from build123d import *

# Parameters (mm, degrees)
F0_W           = 116
F0_H           = 90
F1_DEPTH       = 15
F2_SIZE        = 0.5
F5_D           = 3
F5_DEPTH       = 8
F5_TIP         = 0.9012909285
F6_D           = 4.2
F6_DEPTH       = 13
F6_TIP         = 1.2618073
F7_D           = 5.5
F7_CBORE_D     = 10
F7_CBORE_DEPTH = 6.5


with BuildPart() as f1:
    # F0 (on Top) → F1 (new body)
    with BuildSketch(Plane.XY):
        with Locations((58, 45)):
            Rectangle(F0_W, F0_H)
    extrude(amount=F1_DEPTH)

    # F2
    f2_edges = [f1.edges().sort_by_distance(p)[0] for p in [
        (0, 45, 15),
        (58, 0, 15),
        (116, 45, 15),
        (58, 90, 15),
        (0, 45, 0),
        (58, 0, 0),
        (116, 45, 0),
        (58, 90, 0),
        (0, 0, 7.5),
        (116, 0, 7.5),
        (116, 90, 7.5),
        (0, 90, 7.5),
    ]]
    chamfer(f2_edges, length=F2_SIZE)

    # F5
    with Locations(Plane.XY.offset(15)):
        with Locations((101, 81), (31, 46), (13, 34), (83, 30)):
            Hole(F5_D / 2, depth=F5_DEPTH)
            with Locations((0, 0, -(F5_DEPTH + F5_TIP / 2))):  # 118° drill point
                Cone(0, F5_D / 2, F5_TIP, mode=Mode.SUBTRACT)

    # F6
    with Locations(Plane(origin=(0, 0, 0), x_dir=(1, 0, 0), z_dir=(0, 0, -1))):
        with Locations((105, -45), (11, -45)):
            Hole(F6_D / 2, depth=F6_DEPTH)
            with Locations((0, 0, -(F6_DEPTH + F6_TIP / 2))):  # 118° drill point
                Cone(0, F6_D / 2, F6_TIP, mode=Mode.SUBTRACT)

    # F7 (through all)
    with Locations(Plane(origin=(0, 0, 0), x_dir=(1, 0, 0), z_dir=(0, 0, -1))):
        with Locations((93.5, -61), (93.5, -31), (22, -40)):
            CounterBoreHole(F7_D / 2, F7_CBORE_D / 2, F7_CBORE_DEPTH)


solid = f1.part
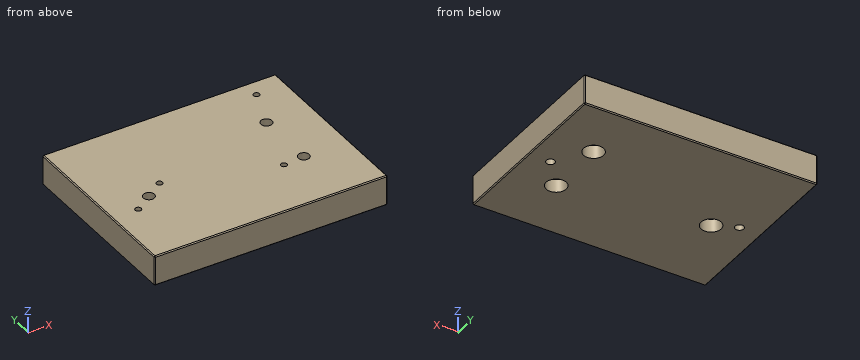
Here's how the part is built. I have some questions about the finished solid (model axes, mm). Coordinates: 2 decimals unless noted, no trailing zeros. Order: outer loops, then holes, each group sorted by start corner. A loop starts at its lowest first (then second) coordinate and runs counter-clockwise, first axis right, second up.
Item 1: I need wall thicknesses on line 1 (Y direction, x = 93.5, z = 2.75); line 2 (X direction, y = 61, z = 3.5); line 3 (Y direction, x = 31, z = 11.5). Which ranges of each line are inside material? Lowest first, please.
Result sheet:
line 1: y = 0 to 26, 36 to 56, 66 to 90
line 2: x = 0 to 88.5, 98.5 to 116
line 3: y = 0 to 44.5, 47.5 to 90
Item 2: If we section it at A-A on y = 61: List the corners of the cut face in (x, z) for me, plus the area to 3 significant figures.
Result sheet:
outline: (0, 0.5) - (0.5, 0) - (88.5, 0) - (88.5, 6.5) - (90.75, 6.5) - (90.75, 15) - (0.5, 15) - (0, 14.5) - close; (96.25, 6.5) - (98.5, 6.5) - (98.5, 0) - (115.5, 0) - (116, 0.5) - (116, 14.5) - (115.5, 15) - (96.25, 15) - close
area: 1,630 mm2
Item 3: For P1, Ø9, axis at x = 22, y = 40, coming from the -Z side, with a flat end and sliding along its axis, tell me the tip position at first contact or that it passes through.
Result sheet:
P1: stops at z = 6.5
